Geometry: see drawing. Coordinates: mm, zero at the bounding-box minimum. Coordinates: 2 decimals unless noted, no trailing zeros. Write each loop counter-clockwise with the first axis right and the second up, starting at its lowest first coordinate (ties: lowest second). Pieces come first, ordered by that corner, then holes. Notation, with made-up numbers: (-34.75, 68) - (-8.75, 68) arc R29 cw to (-8.75, 100) - close; hole circle Ø2 at (26.25, 20). An arc over 180 degrees is marked (long way). Use a Markdown table: item, result. Add a question column.
Q1. Section query B-B (z = 6.5). Return the cut outline in (x, y), then the cut area to 3 significant figures.
Q2. Section query D-D (y = 2.25). Return the cut outline in (x, z) (3 decimals).
Q3. Section query A-A (x = 32.5). Return the cut outline in (y, z), then the cut area to 3 significant figures.
Q4. Mould query, pull axis X, two halves, no side actions, for the marked faces 1, 2, 3 and 4. Classes: released by +X, released by -X, zero draft, split by the parting line, or undercut.
Q5. Material intervals for probe 1 along Z at (x, y) = (32.5, 7.5); probe 2 along Z at (x, y) = (32.5, 10.8); probe 3 along Z at (x, y) = (34, 6) (1 decimal), sorted ascending. Write a range as from..to.
Q6. Pin query (flat end, axial travel): P1, Ø18.5, axis at x = 33.5, z = 48, coming from the +Y side; P2, Ø1, axis at y = 7, z = 26, coming from the +X side; P3, Ø6, axis at x = 38.5, y = 2.5, coming from the -Z side. Return the tip coordinate at first contact, or that it passes through.
Q7. Section query C-C (x = 43.5). Return the cut outline in (y, z).
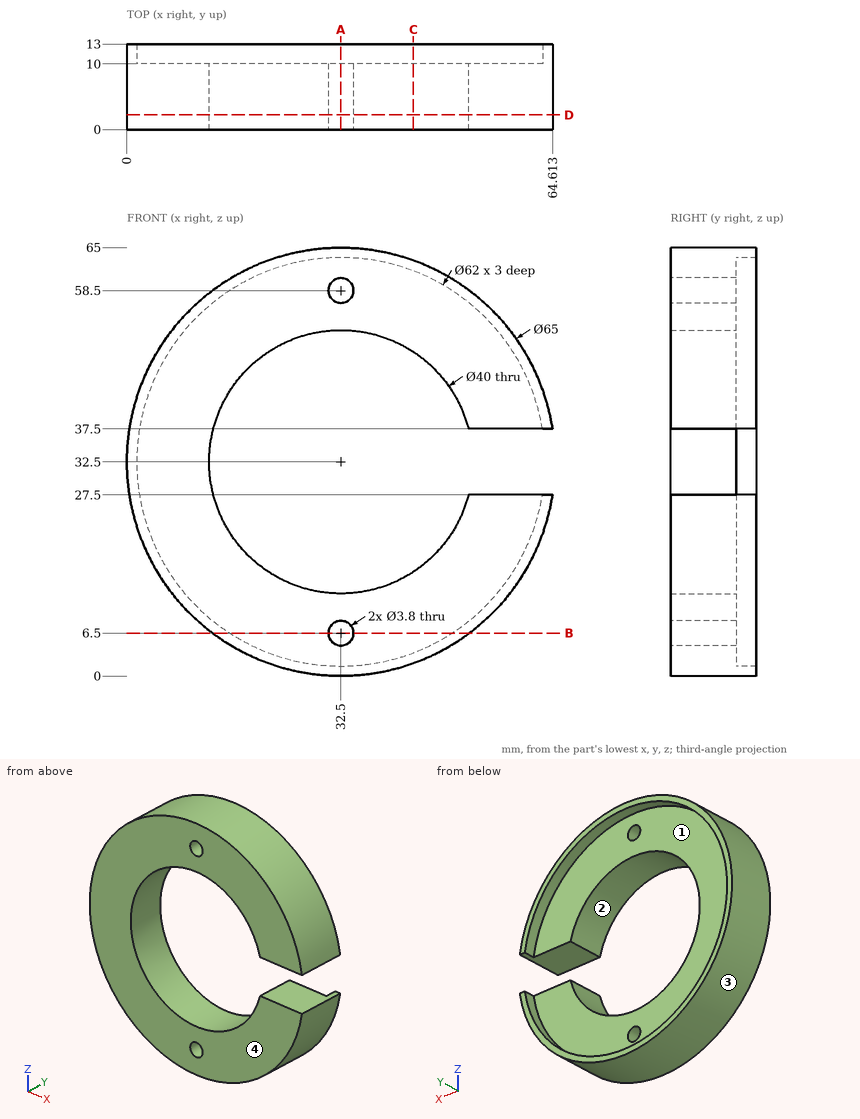
Values follow:
| question | item | result |
|---|---|---|
| 1 | outline | (13, 0) - (30.6, 0) - (30.6, 10) - (15.62, 10) - (15.62, 13) - (13, 13) - close; (34.4, 0) - (52, 0) - (52, 13) - (49.38, 13) - (49.38, 10) - (34.4, 10) - close |
| 1 | area | 368 mm2 |
| 2 | outline | (51.865, 27.5) arc R20 cw (long way) to (51.865, 37.5) - (64.613, 37.5) arc R32.5 ccw (long way) to (64.613, 27.5) - close; hole circle Ø3.8 at (32.5, 6.5); hole circle Ø3.8 at (32.5, 58.5) |
| 3 | outline | (0, 0) - (13, 0) - (13, 1.5) - (10, 1.5) - (10, 4.6) - (0, 4.6) - close; (0, 8.4) - (10, 8.4) - (10, 12.5) - (0, 12.5) - close; (0, 52.5) - (10, 52.5) - (10, 56.6) - (0, 56.6) - close; (0, 60.4) - (10, 60.4) - (10, 63.5) - (13, 63.5) - (13, 65) - (0, 65) - close |
| 3 | area | 183 mm2 |
| 4 | face 1 | undercut |
| 4 | face 2 | undercut |
| 4 | face 3 | split by the parting line |
| 4 | face 4 | zero draft |
| 5 | probe 1 | 0..4.6, 8.4..12.5, 52.5..56.6, 60.4..65 |
| 5 | probe 2 | 0..1.5, 63.5..65 |
| 5 | probe 3 | 0..5.3, 7.7..12.6, 52.4..57.3, 59.7..65 |
| 6 | P1 | y = 10 |
| 6 | P2 | x = 64.44 |
| 6 | P3 | z = 0.14 |
| 7 | outline | (0, 1.92) - (13, 1.92) - (13, 3.52) - (10, 3.52) - (10, 15.8) - (0, 15.8) - close; (0, 49.2) - (10, 49.2) - (10, 61.48) - (13, 61.48) - (13, 63.08) - (0, 63.08) - close |
